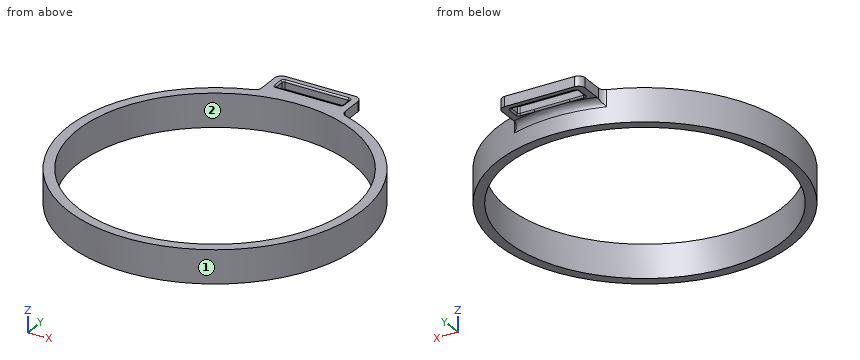
```python
from build123d import *

# Parameters (mm, degrees)
F0_R     = 44.25
F1_DEPTH = 10
F2_R     = 41.25
F3_DEPTH = 15
F5_DEPTH = 3
F6_W     = 20
F6_H     = 4
F7_DEPTH = 25
F8_R     = 2
F9_R     = 0.5


with BuildPart() as f1:
    # F0 (on Top) → F1 (new body)
    with BuildSketch(Plane.XY):
        Circle(F0_R)
    extrude(amount=F1_DEPTH)

    # F2 (on face) → F3 (cut)
    with BuildSketch(Plane.XY.offset(10)):
        Circle(F2_R)
    extrude(amount=-F3_DEPTH, mode=Mode.SUBTRACT)

    # F4 (on face) → F5 (join)
    with BuildSketch(Plane.XY.offset(10)):
        with BuildLine():
            Line((12.5, 52.447762014), (-12.5, 52.447762014))
            Line((-12.5, 52.447762014), (-12.5, 42.447762014))
            ThreePointArc((-12.5, 42.447762014), (0, 44.25), (12.5, 42.447762014))
            Line((12.5, 42.447762014), (12.5, 52.447762014))
        make_face()
    extrude(amount=-F5_DEPTH)

    # F6 (on face) → F7 (cut)
    with BuildSketch(Plane.XY.offset(10)):
        with Locations((0, 48.447762014)):
            Rectangle(F6_W, F6_H)
    extrude(amount=-F7_DEPTH, mode=Mode.SUBTRACT)

    # F8
    f8_edges = [f1.edges().sort_by_distance(p)[0] for p in [
        (0, 44.25, 7),
        (12.5, 42.447762, 8.5),
        (12.5, 52.447762, 8.5),
        (-12.5, 42.447762, 8.5),
        (-12.5, 52.447762, 8.5),
    ]]
    fillet(f8_edges, radius=F8_R)

    # F9
    f9_edges = [f1.edges().sort_by_distance(p)[0] for p in [
        (0, 46.447762, 10),
        (10, 46.447762, 8.5),
        (0, 46.447762, 7),
        (-10, 46.447762, 8.5),
        (-10, 48.447762, 10),
        (-10, 48.447762, 7),
        (-10, 50.447762, 8.5),
        (0, 50.447762, 10),
        (0, 50.447762, 7),
        (10, 50.447762, 8.5),
        (10, 48.447762, 10),
        (10, 48.447762, 7),
    ]]
    fillet(f9_edges, radius=F9_R)


solid = f1.part
```
For this review, take the finished solid that the model builds, in its own axes (mm). Face numbers are marked on the shaded views. Round coordinates to 2 decimals unless told otherwise and drop trailing zeros. Write each loop counter-clockwise with the first axis right and the second up, starting at its lowest first coordinate (ties: lowest second). Pieces come first, ordered by that corner, then holes. Notation, with made-up numbers: (62, 87.5) - (101, 87.5) arc R18 ccw to (101, 106.5) - close; hole circle Ø10 at (18.25, 40). An arc over 180 degrees is marked (long way). Write each question's results on one line, items separated by ' | '.
Item 1: Take a section at B-B on x = 35.5. State the section outline as (y, z) points.
Calculated:
outline: (-26.42, 0) - (-21.01, 0) - (-21.01, 10) - (-26.42, 10) - close; (21.01, 0) - (26.42, 0) - (26.42, 10) - (21.01, 10) - close
Item 2: Take a section at C-C on z = 3.5. State the section outline as (x, y) points.
Calculated:
outline: circle Ø88.5 at (0, 0); hole circle Ø82.5 at (0, 0)
Item 3: Draft analysis for pull direction X (two halves, no side actions). For the marked faces 1 and 2, state which applies: pulls with the +X half, pulls with the -X half, needs draft (parallel to the pull), parting line crosses it, or undercut.
Calculated:
face 1: parting line crosses it | face 2: undercut
Item 4: Take a section at A-A on y = 0. State the section outline as (x, z) points.
Calculated:
outline: (-44.25, 0) - (-41.25, 0) - (-41.25, 10) - (-44.25, 10) - close; (41.25, 0) - (44.25, 0) - (44.25, 10) - (41.25, 10) - close
Item 5: Take a section at D-D on x = 0. Count the separate pieces of the cut face and the enclosed holes in it, then the cut area to 3 significant figures.
Calculated:
separate pieces: 3 | enclosed holes: 0 | area: 73.2 mm^2
Item 6: For pin 1 (1 mm diameter, centred on x = 1.5, z = 8.5, fed in from -Y); pin 2 (5 mm diameter, centred on x = 32, z = 7, fed in from +Y); pin 3 (1.5 mm diameter, centred on x = 11, z = 1, fed in from +Y), all flat-tipped, find the tip position at first contact; note any pin that passes through.
Calculated:
pin 1: stops at y = -44.24 | pin 2: stops at y = 32.98 | pin 3: stops at y = 43.05
Item 7: To check wall thickness, follow line 1 along Y through (x, z) = (0, 3.5); line 2 along X through (y, z) = (23, 2.75); line 3 along X through (y, z) = (24, 9.25). State the ranges of each line that lie inside material, in increasing order. Write a range as from..to.
Calculated:
line 1: y = -44.25..-41.25, 41.25..44.25 | line 2: x = -37.8..-34.24, 34.24..37.8 | line 3: x = -37.18..-33.55, 33.55..37.18
